Verification items for the finished model (mm, model axes). A direction names the side the tool comes from. Coordinates: 2 decimals unless noted, no trailing zeros. Write each loop counter-clockwise with the first axis right and the second up, starting at its lowest first coordinate (ties: lowest second). Pieces come first, ordered by that corner, then holes.
```python
from build123d import *

# Parameters (mm, degrees)
SKETCH1_R           = 63.5
BOSS_EXTRUDE1_DEPTH = 38.1
SKETCH2_R           = 57.15
CUT_EXTRUDE4_DEPTH  = 40.64
SKETCH4_W           = 2.772986199
SKETCH4_H           = 2.54
CUT_EXTRUDE7_DEPTH  = 40.64
CIRPATTERN1_COUNT   = 40


with BuildPart() as part:
    # Sketch1 → Boss-Extrude1 (new body)
    with BuildSketch(Plane(origin=(0, 0, 0), x_dir=(0, 0, -1), z_dir=(1, 0, 0))):
        with Locations(Location((0, 0, 0), (0, 0, 180))):
            Circle(SKETCH1_R)
    extrude(amount=BOSS_EXTRUDE1_DEPTH)

    # Sketch2 → Cut-Extrude4 (cut)
    with BuildSketch(Plane(origin=(0, 0, 0), x_dir=(0, 0, -1), z_dir=(1, 0, 0))):
        Circle(SKETCH2_R)
    extrude(amount=CUT_EXTRUDE4_DEPTH, mode=Mode.SUBTRACT)

    # Sketch4 → Cut-Extrude7 (cut)
    with BuildSketch(Plane.ZY):
        with Locations((-62.113506901, -1.27)):
            Rectangle(SKETCH4_W, SKETCH4_H)
    cut_extrude7 = extrude(amount=-CUT_EXTRUDE7_DEPTH, mode=Mode.SUBTRACT)

    # CirPattern1: Cut-Extrude7 ×40 about axis
    cirpattern1_axis = Axis((0, 0, 0), (1, 0, 0))
    for i in range(1, CIRPATTERN1_COUNT):
        add(cut_extrude7.rotate(cirpattern1_axis, i * 360 / CIRPATTERN1_COUNT), mode=Mode.SUBTRACT)


solid = part.part
```
1. Gauge pin test, flat ends, axial feed: P1, Ø3, axis at x = 17, z = -62, coming from the +Y side; P2, Ø12, axis at x = 31, y = -28, coming from the -Z side; P3, Ø3, axis at x = 13.5, z = -46.5, coming from the -Y side. Record the tip position at first contact, or that the pin passes through.
2. Material ranges on L1, parallel to Y at x = 35, z = -38.5; L2, parallel to Y at x = 12.5, z = 6.5; L3, parallel to Z at x = 10, y = -27, recorded low to high.
3. Tool access check on faces 1 (the cylindrical face through (18.783, 61.423, -16.106)), 2 (the flat face through (19, 62, 0)). Record the directions out of +Z, -Z, +X, -X, +Y, -Y that give a thin tool (end or side, any length) a straight path to the whole face; none if there is none.
4. Sectioned sample at A-A, the plane z = -5. Record the boundary of the cut face in (x, y), and give its area (3 significant figures).
5. Draft check along Y on faces 3 (the cylindrical face through (18.783, -63.187, 6.299)), 4 (the cylindrical face through (18.78, 49.13, 40.23)), 5 (the flat face through (19, 0, 62)). Enter one of: pulls with the +Y half, pulls with the -Y half, needs draft (parallel to the pull), parting line crosses it, or undercut.
Outcome:
1. P1: stops at y = 17.19
1. P2: stops at z = -59.56
1. P3: stops at y = -44.8
2. L1: y = -50.5 to -42.24, 42.24 to 48.67
2. L2: y = -63.17 to -56.78, 56.78 to 63.17
2. L3: z = -57.47 to -50.37, 50.37 to 54.4
3. face 1: -Z, +X, -X, +Y
3. face 2: +X, -X, +Y
4. outline: (0, -63.3) - (38.1, -63.3) - (38.1, -56.93) - (0, -56.93) - close; (0, 56.93) - (38.1, 56.93) - (38.1, 63.3) - (0, 63.3) - close
4. area: 486 mm2
5. face 3: pulls with the -Y half
5. face 4: pulls with the +Y half
5. face 5: undercut
